from build123d import *

# Parameters (mm, degrees)
SCHIZZO2_W                   = 150
SCHIZZO2_H                   = 150
ESTRUSIONE_ESTRUSIONE1_DEPTH = 5
SCHIZZO3_W                   = 50
SCHIZZO3_H                   = 15
ESTRUSIONE_ESTRUSIONE2_DEPTH = 95
SCHIZZO6_R                   = 5
ESTRUSIONE_ESTRUSIONE3_DEPTH = 61.630141236


with BuildPart() as part:
    # Schizzo2 → Estrusione-Estrusione1 (new body)
    with BuildSketch(Plane.XY):
        with Locations((75, 75)):
            Rectangle(SCHIZZO2_W, SCHIZZO2_H)
    extrude(amount=-ESTRUSIONE_ESTRUSIONE1_DEPTH)

    # Schizzo3 → Estrusione-Estrusione2 (add)
    with BuildSketch(Plane.XY):
        with Locations((74.643012927, 47.5)):
            Rectangle(SCHIZZO3_W, SCHIZZO3_H)
        with Locations((75, 102.5)):
            Rectangle(SCHIZZO3_W, SCHIZZO3_H)
    extrude(amount=ESTRUSIONE_ESTRUSIONE2_DEPTH)

    # Schizzo6 → Estrusione-Estrusione3 (add)
    with BuildSketch(Plane.XZ.offset(-40)):
        with Locations(Location((74.643012927, 70, 0), (0, 0, 270))):
            Circle(SCHIZZO6_R)
    extrude(amount=-ESTRUSIONE_ESTRUSIONE3_DEPTH)


solid = part.part
Check sheet for the modelled part. Datum: model origin and axes. Units: mm. A direction names the side the tool comes from. Coordinates: 2 decimals unless noted, no trailing zeros. Write each loop counter-clockwise with the first axis right and the second up, starting at its lowest first coordinate (ties: lowest second). Pieces come first, ordered by that corner, then holes.
Item 1: Cross-section at D-D on y = 88.5. Record the boundary of the cut face in (x, z).
Numbers:
outline: (0, -5) - (150, -5) - (150, 0) - (0, 0) - close; circle Ø10 at (74.64, 70)
Item 2: Depth check by flat-ended pin: pin 1 Ø7.5 at (y, z) = (51, 40) entering from +X; pin 2 Ø6 at (x, z) = (76, 36.5) entering from -Y; pin 3 Ø6 at (x, z) = (81, 10.5) entering from +Y. Enter the tip coordinate at first touch or a pass-through.
Numbers:
pin 1: stops at x = 99.64
pin 2: stops at y = 40
pin 3: stops at y = 110
Item 3: Cross-section at C-C on z = 70. Record the boundary of the cut face in (x, y), then the cut area to 3 significant figures.
Numbers:
outline: (49.64, 40) - (99.64, 40) - (99.64, 55) - (79.64, 55) - (79.64, 95) - (100, 95) - (100, 110) - (50, 110) - (50, 95) - (69.64, 95) - (69.64, 55) - (49.64, 55) - close
area: 1,900 mm2
Item 4: Cross-section at A-A on z = 43.5. Record the boundary of the cut face in (x, y).
Numbers:
outline: (49.64, 40) - (99.64, 40) - (99.64, 55) - (49.64, 55) - close; (50, 95) - (100, 95) - (100, 110) - (50, 110) - close
Item 5: Scan lines: probe 1 along Y at (x, z) = (98, 14.5); probe 2 along Z at (x, y) = (45.5, 76); probe 3 along X at (y, z) = (49.5, 84). Record each from-to range of solid material in increasing order.
Numbers:
probe 1: y = 40 to 55, 95 to 110
probe 2: z = -5 to 0
probe 3: x = 49.64 to 99.64
Item 6: Access from +Z, -Z, +X, -X, +Y, -Y to the whole of each face (thin tool, end or side, straight path). Record for faces 4 (the face through (99.643, 47, 47)), 5 (the face through (100, 102, 47)), 6 (the face through (78.86, 74.72, 67.31)).
Numbers:
face 4: +Z, +X, -Y
face 5: +Z, +X, +Y, -Y
face 6: none
Item 7: Cross-section at B-B on y = 105. Record the boundary of the cut face in (x, z).
Numbers:
outline: (0, -5) - (150, -5) - (150, 0) - (100, 0) - (100, 95) - (50, 95) - (50, 0) - (0, 0) - close
Item 8: Mould release check, pull along Y, two halves, no side actions. Record for faces 1 (the face through (74, 0, -2)), 2 (the face through (74, 55, 47)), 3 (the face through (0, 74, -2)): released by +Y, released by -Y, zero draft, split by the parting line, or undercut.
Numbers:
face 1: released by -Y
face 2: undercut
face 3: zero draft
